```python
from build123d import *

# Parameters (mm, degrees)
F0_R     = 12.5
F0_R_2   = 2.5
F1_DEPTH = 2
F2_R     = 1
F3_R     = 0.99999


# Not quite as in the source:
# - a fillet or chamfer is up to 0.001 mm smaller than in the source, because OpenCascade refuses the exact size


with BuildPart() as f1:
    # F0 (on Top) → F1 (new body)
    with BuildSketch(Plane.XY):
        Circle(F0_R)
        Circle(F0_R_2, mode=Mode.SUBTRACT)
    extrude(amount=F1_DEPTH)

    # F2
    f2_edges = [f1.edges().sort_by_distance(p)[0] for p in [
        (-12.5, 0, 2),
    ]]
    fillet(f2_edges, radius=F2_R)

    # F3 (radius 1 in the source; OpenCascade refuses exactly that, so slightly less here)
    f3_edges = [f1.edges().sort_by_distance(p)[0] for p in [
        (-12.5, 0, 0),
    ]]
    fillet(f3_edges, radius=F3_R)


solid = f1.part
```
Check sheet for the modelled part. Datum: model origin and axes. Units: mm. Give positions to 0.01 mm unless a question says otherwise; leave off trailing zeros. Order: outer loops, then holes, each group sorted by start corner. A loop starts at its lowest first (then second) coordinate and runs counter-clockwise, first axis right, second up. Notation, with made-up numbers: M -37.75,24 L -2.75,24 A19 ccw -2.75,52 Z; hole C 2,80.25 d2. An arc over 180 degrees is marked long. Answer in a Markdown table with one row per item. Add a question column.
Q1. Gauge pin test, flat ends, axial feed: pin 1 Ø8 at (x, y) = (4.5, -4.5) entering from -Z; pin 2 Ø1 at (y, z) = (6.5, 1) entering from -X. Record the tip position at first contact, or that the pin passes through.
Q2. Sectioned sample at C-C, the plane z = 1.4. Record the boundary of the cut face in (x, y), and give its area (3 significant figures).
Q3. Thickness scan on L1, parallel to Y at x = 0, z = 0.95; L2, parallel to Y at x = -2, z = 1.8; L3, parallel to X at y = 1.75, z = 0.45. Record the ranges inside material, lowest first.
Q4. Release check for a two-part mould opening along X. For faces 1 (the flat face through (0, 3, 0)), 2 (the cylindrical face through (-0.54, -2.44, 0.99)) record: released by +X, released by -X, zero draft, split by the parting line, or undercut.
Verdict:
| question | item | result |
|---|---|---|
| 1 | pin 1 | z = 0 |
| 1 | pin 2 | x = -10.97 |
| 2 | outline | C 0,0 d24.83; hole C 0,0 d5 |
| 2 | area | 465 mm² |
| 3 | L1 | -12.5 to -2.5, 2.5 to 12.5 |
| 3 | L2 | -11.93 to -1.5, 1.5 to 11.93 |
| 3 | L3 | -12.21 to -1.79, 1.79 to 12.21 |
| 4 | face 1 | zero draft |
| 4 | face 2 | undercut |
